Check sheet for the drawn part. Datum: minimum x, y, z corner. Units: mm. A direction names the side the tool comes from. Coordinates: 2 decimals unless noted, no trailing zeros. Write each loop counter-clockwise with the first axis right and the second up, starting at its lowest first coordinate (ties: lowest second). Pieces come first, ordered by that corner, then holes. Notation, with made-up numbers: M 38.25,-39 L 45.25,-39 A17 cw 45.25,-26 Z; hole C 22.5,-34 d2. An arc over 180 degrees is marked long. Answer in a Markdown table with one row per item.
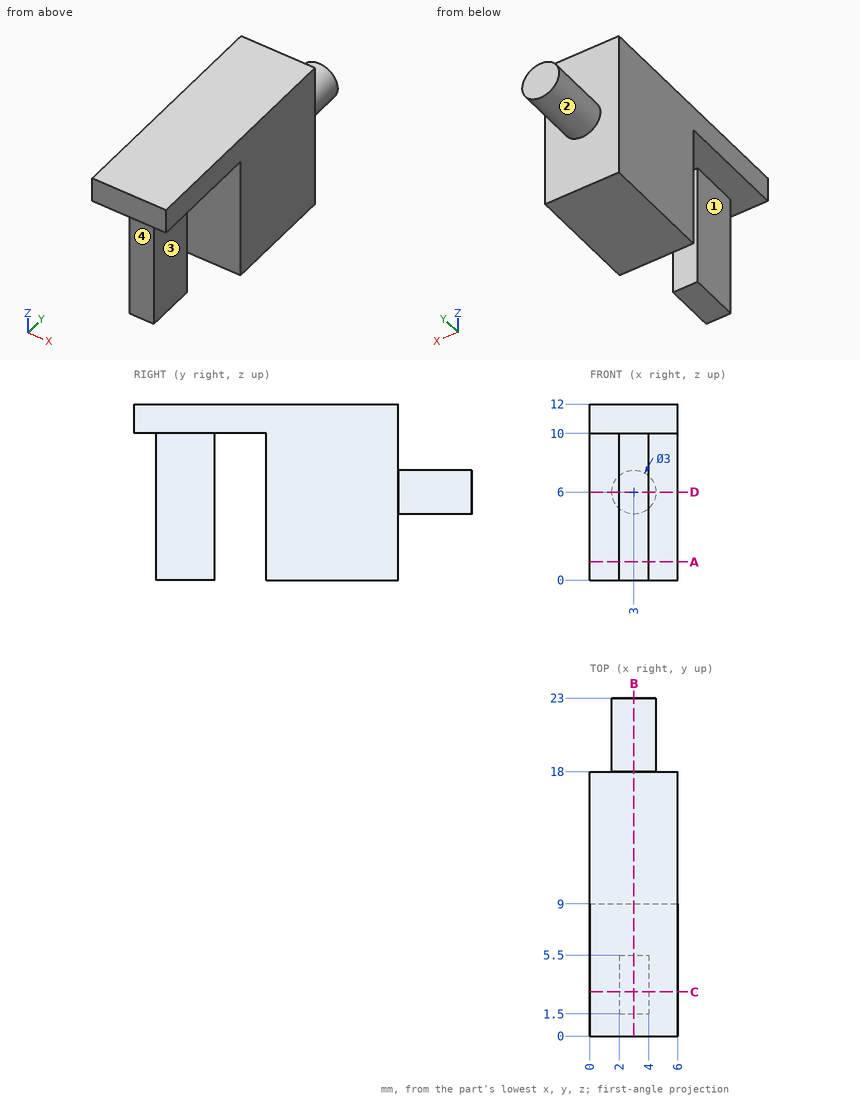
1) Sectioned sample at B-B (x = 3). Record the cut outline in (y, z).
Response values:
| item | result |
|---|---|
| outline | M 0,10 L 1.5,10 L 1.5,0 L 5.5,0 L 5.5,10 L 9,10 L 9,0 L 18,0 L 18,4.5 L 23,4.5 L 23,7.5 L 18,7.5 L 18,12 L 0,12 Z |
2) Thickness scan on L1, parallel to Y at x = 2.8, z = 7; L2, parallel to Y at x = 3.9, z = 3; L3, parallel to Z at x = 0.3, y = 8. Record the ranges inside material, lowest first. Write a range as [from, to].
Response values:
| item | result |
|---|---|
| L1 | y = [1.5, 5.5], [9, 23] |
| L2 | y = [1.5, 5.5], [9, 18] |
| L3 | z = [10, 12] |
3) Sectioned sample at C-C (y = 3). Record the cut outline in (x, z).
Response values:
| item | result |
|---|---|
| outline | M 0,10 L 2,10 L 2,0 L 4,0 L 4,10 L 6,10 L 6,12 L 0,12 Z |
4) Depth check by flat-ended pin: pin 1 (4.5 mm diameter, centred on y = 3, z = 6.5, fed in from -X); pin 2 (2 mm diameter, centred on x = 2.5, z = 3, fed in from +Y); pin 3 (1.5 mm diameter, centred on x = 1.5, y = 19.5, fed in from -Z). Enter the tip coordinate at first touch or a pass-through.
Response values:
| item | result |
|---|---|
| pin 1 | stops at x = 2 |
| pin 2 | stops at y = 18 |
| pin 3 | stops at z = 4.7 |
5) Sectioned sample at A-A (z = 1.25). Record the cut outline in (x, y).
Response values:
| item | result |
|---|---|
| outline | M 0,9 L 6,9 L 6,18 L 0,18 Z; M 2,1.5 L 4,1.5 L 4,5.5 L 2,5.5 Z |
6) Tool access check on the marked faces 1, 2, 3 and 4. Record the directions out of +Z, -Z, +X, -X, +Y, -Y that give a thin tool (end or side, any length) a straight path to the whole face; none if there is none.
Response values:
| item | result |
|---|---|
| face 1 | -Z, -X, -Y |
| face 2 | +Y |
| face 3 | -Z, +X, -Y |
| face 4 | -Z, +X, -X, -Y |
7) Sectioned sample at D-D (z = 6). Record the cut outline in (x, y).
Response values:
| item | result |
|---|---|
| outline | M 0,9 L 6,9 L 6,18 L 4.5,18 L 4.5,23 L 1.5,23 L 1.5,18 L 0,18 Z; M 2,1.5 L 4,1.5 L 4,5.5 L 2,5.5 Z |
